Part model, mm, in its own coordinate system. Give positions to 0.01 mm unless a question says otherwise; leave off trailing zeros. Write each loop counter-clockwise with the first axis right and the second up, starting at its lowest first coordinate (ties: lowest second). Pieces come first, ordered by that corner, then holes.
Autodesk Inventor part; units mm, degrees
ref_plane "YZ Plane" through (0, 0, 0) normal (1, 0, 0) x (0, 1, 0)
ref_plane "XZ Plane" through (0, 0, 0) normal (0, 1, 0) x (-1, 0, 0)
ref_plane "XY Plane" through (0, 0, 0) normal (0, 0, 1) x (1, 0, 0)
sketch "スケッチ1" plane through (0, 0, 0) normal (0, 1, 0) x (-1, 0, 0)
  line L0 (0, 0) -> (-40, 0)
  line L1 (-40, 0) -> (-40, -115)
  line L2 (-40, -115) -> (0, -115)
  line L3 (0, -115) -> (0, 0)
  dimension "d0" = 40
  dimension "d1" = 115
extrude "押し出し1" add sketch "スケッチ1" along normal blind 3
sketch "スケッチ2" plane through (0, 3, 0) normal (0, 1, 0) x (1, 0, 0)
  line L0 (0, 0) -> (40, 0) construction
  line L1 (20, 0) -> (20, 115) construction
  line L2 (40, 115) -> (0, 115) construction
  point P0 (20, 18)
  dimension "d4" = 18
hole "穴1" at (20, 3, -18) direction (0, -1, 0) diameter 8.5 end through all
sketch "スケッチ3" plane through (0, 3, 0) normal (0, 1, 0) x (1, 0, 0)
  circle A0 centre (20, 18) radius 4.25 construction
  circle A1 centre (20, 18) radius 12.5 construction
  point P0 (0, 0)
  point P1 (7.5, 18)
  point P2 (20, 5.5)
  point P3 (32.5, 18)
  point P4 (20, 30.5)
  dimension "d12" = 25
  dimension "d15" = 360
hole "穴2" at (7.5, 3, -18) at (20, 3, -5.5) at (32.5, 3, -18) at (20, 3, -30.5) direction (0, -1, 0) diameter 2.459 end through all
sketch "スケッチ4" plane through (0, 3, 0) normal (0, 1, 0) x (1, 0, 0)
  line L0 (40, 115) -> (0, 115) construction
  line L1 (0, 115) -> (40, 115) construction
  line L2 (40, 115) -> (40, 110) construction
  line L3 (40, 110) -> (0, 110) construction
  line L4 (0, 110) -> (0, 115) construction
  line L5 (0, 115) -> (0, 0)
  line L6 (0, 112.5) -> (40, 112.5) construction
  line L7 (40, 0) -> (40, 115)
  line L8 (0, 115) -> (0, 0) construction
  line L9 (40, 85) -> (0, 85) construction
  line L10 (0, 85) -> (0, 90) construction
  line L11 (0, 90) -> (40, 90) construction
  line L12 (40, 90) -> (40, 85) construction
  line L13 (40, 87.5) -> (0, 87.5) construction
  point P0 (4, 112.5)
  point P1 (36, 112.5)
  point P2 (36, 87.5)
  point P3 (4, 87.5)
  dimension "d25" = 5
  dimension "d26" = 4
  dimension "d27" = 4
  dimension "d35" = 5
  dimension "d36" = 25
hole "穴3" [suppressed]
sketch "スケッチ5" plane through (0, 3, 0) normal (0, 1, 0) x (1, 0, 0)
  line L0 (36, 84.5) -> (4, 84.5) construction
  line L1 (4, 84.5) -> (4, 109.5) construction
  line L2 (4, 109.5) -> (36, 109.5) construction
  line L3 (36, 109.5) -> (36, 84.5) construction
  line L4 (40, 0) -> (40, 115) construction
  line L5 (0, 115) -> (0, 0) construction
  line L6 (40, 115) -> (0, 115) construction
  dimension "d37" = 4
  dimension "d38" = 4
  dimension "d39" = 5.5
  dimension "d40" = 25
hole "穴4" at (36, 3, -84.5) at (36, 3, -109.5) at (4, 3, -109.5) at (4, 3, -84.5) direction (0, -1, 0) diameter 2.459 end through all
properties part number "shoulder1_upper_cover" material "アルミニウム 5052"
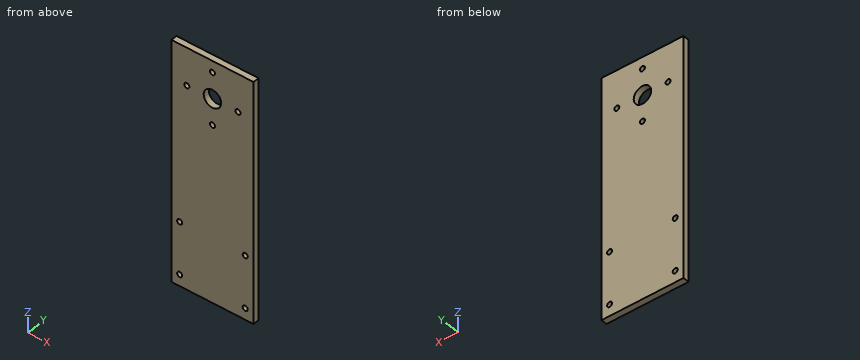
1) Saw through at C-C, the plane z = -84.5. Write the cut outline in (x, y).
Answers follow:
outline: (0, 0) - (2.77, 0) - (2.77, 3) - (0, 3) - close; (5.23, 0) - (34.77, 0) - (34.77, 3) - (5.23, 3) - close; (37.23, 0) - (40, 0) - (40, 3) - (37.23, 3) - close
2) Saw through at B-B, the plane z = -5.5. Write the cut outline in (x, y).
Answers follow:
outline: (0, 0) - (18.77, 0) - (18.77, 3) - (0, 3) - close; (21.23, 0) - (40, 0) - (40, 3) - (21.23, 3) - close
3) Pin check, flat tip, straight feed: pin 1 Ø2 at (x, z) = (32.5, -18) entering from +Y. Stop position of the tip, or through.
Answers follow:
pin 1: passes through
4) Wall check: L1, parallel to X at y = 1.55, z = -109.5; L2, parallel to X at y = 2, z = -18; L3, parallel to Z at x = 36, y = 0.25. Give the ranges that are in metal, low to high.
Answers follow:
L1: x = 0 to 2.77, 5.23 to 34.77, 37.23 to 40
L2: x = 0 to 6.27, 8.73 to 15.75, 24.25 to 31.27, 33.73 to 40
L3: z = -115 to -110.73, -108.27 to -85.73, -83.27 to 0
5) Saw through at D-D, the plane x = 20. Write the cut outline in (y, z), then the cut area to 3 significant figures.
Answers follow:
outline: (0, -115) - (3, -115) - (3, -31.73) - (0, -31.73) - close; (0, -29.27) - (3, -29.27) - (3, -22.25) - (0, -22.25) - close; (0, -13.75) - (3, -13.75) - (3, -6.73) - (0, -6.73) - close; (0, -4.27) - (3, -4.27) - (3, 0) - (0, 0) - close
area: 305 mm2
6) Saw through at A-A, the plane x = 32.5. Write the cut outline in (y, z), then the cut area to 3 significant figures.
Answers follow:
outline: (0, -115) - (3, -115) - (3, -19.23) - (0, -19.23) - close; (0, -16.77) - (3, -16.77) - (3, 0) - (0, 0) - close
area: 338 mm2
